For this review, take the finished solid that the model builds, in its own axes (mm). A direction names the side the tool comes from. Give positions to 0.01 mm unless a question says otherwise; leave off trailing zeros. Write each loop counter-clockwise with the first axis right and the second up, starting at its lowest first coordinate (ties: lowest second). Pieces come first, ordered by that corner, then holes. Notation, with made-up numbers: (37, -25) -> (94, -25) arc R16 cw to (94, -20) -> close; hole circle Ø7 at (-28, 36.5). An arc over 180 degrees is marked (long way). Return JSON: item names as keys, results as strings.
from build123d import *

# Parameters (mm, degrees)
BOSS_EXTRU_5_DEPTH      = 4.5
BOSS_EXTRU_5_DEPTH_BACK = 4.5
CONG_1_R                = 150
CONG_2_R                = 10


with BuildPart() as part:
    # Esquisse1 → Boss.-Extru.5 (new, two sides: drawn at the far end of the back side and taken through both)
    with BuildSketch(Plane.XY.offset(-BOSS_EXTRU_5_DEPTH_BACK)):
        Polygon((0, 0), (-758.779695033, 0), (-957.678777511, 212.988479036), (-957.678777511, 232.988479036), (-878.536330397, 232.988479036), (-878.536330397, 212.988479036), (-875.536330397, 212.988479036), (-875.536330397, 230.940110876), (-827.928204377, 170.423574705), (-795.486560581, 139.307598786), (-795.486560581, 119.307598786), (-792.486560581, 119.307598786), (-792.486560581, 133.699221334), (-727.464635299, 77.5420493), (-605.872801012, 77.5420493), (-605.872801012, 57.5420493), (-602.872801012, 57.5420493), (-602.872801012, 77.5420493), (-221.085552101, 77.5420493), (-221.085552101, 57.5420493), (-218.085552101, 57.5420493), (-218.085552101, 77.5420493), (-202.36477071, 77.5420493), (-66.626684698, 263.704257097), (57.709039867, 296.235629936), (46.096581547, 244.724780595), (49.02313659, 244.06502641), (46.758497819, 234.019481935), (-61.251050758, 91.440931648), (-61.251050758, 23.544195216), (0, 23.544195216), align=None)
    extrude(amount=BOSS_EXTRU_5_DEPTH + BOSS_EXTRU_5_DEPTH_BACK)

    # Cong_1
    cong_1_edges = [part.edges().sort_by_distance(p)[0] for p in [
        (-758.779695033, 0, 0),
    ]]
    fillet(cong_1_edges, radius=CONG_1_R)

    # Cong_2
    cong_2_edges = [part.edges().sort_by_distance(p)[0] for p in [
        (-957.678777511, 212.988479036, 0),
        (-957.678777511, 232.988479036, 0),
    ]]
    fillet(cong_2_edges, radius=CONG_2_R)


solid = part.part
1. For faces 5 (the flat face through (-5.33, 279.74, -0.06)), 6 (the flat face through (-760.431, 106.014, -0.063)), list the 3-axis set-ups (+Z, -Z, +X, -X, +Y, -Y) from which the entire face can be reached by the end or side of a thin tool; tool diameter is ignored.
Results found:
{"face 5": "+Z, -Z, -X, +Y", "face 6": "+Z, -Z, +Y"}
2. Add section A-A, the plane x = -45. State the section outline as (y, z) points, plus the area to 3 significant figures.
Results found:
{"outline": "(0, -4.5) -> (23.54, -4.5) -> (23.54, 4.5) -> (0, 4.5) -> close; (112.89, -4.5) -> (269.36, -4.5) -> (269.36, 4.5) -> (112.89, 4.5) -> close", "area": "1,620 mm²"}
3. For pin 1 (2.5 mm diameter, centred on y = 226, z = 0.5, fed in from -X); pin 2 (0.9 mm diameter, centred on x = -220, z = 2, fed in from +Y); pin 3 (2 mm diameter, centred on x = -79, z = -3.5, fed in from +Y); pin 4 (3 mm diameter, centred on x = -479, z = -2.5, fed in from -Y), all flat-tipped, find the tip position at first contact; note any pin that passes through.
Results found:
{"pin 1": "stops at x = -957.52", "pin 2": "stops at y = 57.54", "pin 3": "stops at y = 248.11", "pin 4": "stops at y = 0"}
4. To check wall thickness, follow probe 1 along X at (y, z) = (220, 0); probe 2 along X at (y, z) = (229.5, -1.5); probe 3 along X at (y, z) = (149.5, 3.75). State the ranges of each line that lie inside material, in increasing order.
Results found:
{"probe 1": "x = -957.68 to -878.54, -875.54 to -866.93, -98.49 to 36.14", "probe 2": "x = -955.27 to -878.54, -875.54 to -874.4, -91.57 to 43.33", "probe 3": "x = -898.39 to -806.11, -149.9 to -17.27"}
5. Add section C-C, the plane x = -387. State the section outline as (y, z) points, plus the area to 3 significant figures.
Results found:
{"outline": "(0, -4.5) -> (77.54, -4.5) -> (77.54, 4.5) -> (0, 4.5) -> close", "area": "698 mm²"}
6. Add section D-D, the plane x = -853.5. State the section outline as (y, z) points, plus the area to 3 significant figures.
Results found:
{"outline": "(101.43, -4.5) -> (202.93, -4.5) -> (202.93, 4.5) -> (101.43, 4.5) -> close", "area": "913 mm²"}
7. The part is to be moulded in two halves that separate along Y. For faces 1 (the flat face through (-6.49, 163.73, -0.06)), 2 (the flat face through (-852.07, 201.11, -0.06)), 3 (the flat face through (-410, 61, -4.5)), 4 (the cylindrical face through (-752.594, 12.079, 0.063)), say which applies: +Y half, -Y half, draft (parallel to the pull), parting line (faces both ways), or undercut.
Results found:
{"face 1": "undercut", "face 2": "+Y half", "face 3": "draft", "face 4": "-Y half"}
